Source: CAD feature listing. Evaluate the final solid. Frame: model axes, mm. A direction names the side the tool comes from. Give positions to 0.01 mm unless a question says otherwise; leave off trailing zeros. Loops run counter-clockwise (first coordinate to the right, second up) from the corner with the lowest first, then second, coordinate; pieces in that order, holes last.
```python
from build123d import *

# Parameters (mm, degrees)
SKETCH1_R            = 44.45
SKETCH1_R_2          = 36
BOSS_EXTRUDE1_DEPTH  = 3
SKETCH1_3_R          = 36
SKETCH1_3_R_2        = 32.5
BOSS_EXTRUDE2_DEPTH  = 2
M3_CLEARANCE_HOLE1_D = 3.2
CIRPATTERN1_COUNT    = 5


with BuildPart() as part:
    # Sketch1 → Boss-Extrude1 (new body)
    with BuildSketch(Plane(origin=(0, 0, 0), x_dir=(1, 0, 0), z_dir=(0, 1, 0))):
        with Locations(Location((0, 0, 0), (0, 0, 270))):
            Circle(SKETCH1_R)
        with Locations(Location((0, 0, 0), (0, 0, 270))):
            Circle(SKETCH1_R_2, mode=Mode.SUBTRACT)
    extrude(amount=BOSS_EXTRUDE1_DEPTH)

    # Sketch1_3 → Boss-Extrude2 (add)
    with BuildSketch(Plane(origin=(0, 0, 0), x_dir=(1, 0, 0), z_dir=(0, 1, 0))):
        with Locations(Location((0, 0, 0), (0, 0, 270))):
            Circle(SKETCH1_3_R)
        with Locations(Location((0, 0, 0), (0, 0, 270))):
            Circle(SKETCH1_3_R_2, mode=Mode.SUBTRACT)
    extrude(amount=BOSS_EXTRUDE2_DEPTH)

    # M3 Clearance Hole1 (through all)
    with Locations(Plane(origin=(0, 3, 0), x_dir=(1, 0, 0), z_dir=(0, 1, 0))):
        with Locations((-41.5, 0)):
            m3_clearance_hole1 = Hole(M3_CLEARANCE_HOLE1_D / 2)

    # CirPattern1: M3 Clearance Hole1 ×5 about axis
    cirpattern1_axis = Axis((0, 0, 0), (0, 1, 0))
    for i in range(1, CIRPATTERN1_COUNT):
        add(m3_clearance_hole1.rotate(cirpattern1_axis, i * 360 / CIRPATTERN1_COUNT), mode=Mode.SUBTRACT)


solid = part.part
```
(1) Section B-B, the plane z = 0. Return the cut outline in (x, y).
A:
outline: (-44.45, 0) - (-43.1, 0) - (-43.1, 3) - (-44.45, 3) - close; (-39.9, 0) - (-32.5, 0) - (-32.5, 2) - (-36, 2) - (-36, 3) - (-39.9, 3) - close; (32.5, 0) - (44.45, 0) - (44.45, 3) - (36, 3) - (36, 2) - (32.5, 2) - close
(2) Section C-C, the plane y = 2.5. Return the cut outline in (x, z).
A:
outline: circle Ø88.9 at (0, 0); hole circle Ø3.2 at (-41.5, 0); hole circle Ø72 at (0, 0); hole circle Ø3.2 at (-12.82, -39.47); hole circle Ø3.2 at (-12.82, 39.47); hole circle Ø3.2 at (33.57, -24.39); hole circle Ø3.2 at (33.57, 24.39)
(3) Ray query, line 1 along X through (y, z) = (0.85, 23); line 2 along X through (y, z) = (0.85, 25); line 3 along X through (y, z) = (2.25, -6.5). Return the intervals inside material, ascending.
A:
line 1: x = -38.04 to -22.96, 22.96 to 32.79, 34.36 to 38.04
line 2: x = -36.75 to -20.77, 20.77 to 32.09, 35.05 to 36.75
line 3: x = -43.97 to -35.41, 35.41 to 43.97
(4) Mould query, pull axis Z, two halves, no side actions, for faces 1 (the flat face through (-36, 3, -4)), 2 (the cylindrical face through (37.48, 1.48, 23.9)), 3 (the cylindrical face through (9.76, 0.99, 31)). Classes: pulls with the +Z half, pulls with the -Z half, needs draft (parallel to the pull), parting line crosses it, or undercut.
A:
face 1: needs draft
face 2: parting line crosses it
face 3: undercut
(5) First-contact query: pin 1 (1.5 mm diameter, centred on y = 1.5, z = 27.5, fed in from +X); pin 2 (1 mm diameter, centred on x = -11.5, y = 1.5, fed in from +Z). Flat tips, straight axial feed; report the tip coordinate or a pass-through.
A:
pin 1: stops at x = 35.5
pin 2: stops at z = 43.07
(6) Reachability of faces 4 (the cylindrical face through (10.81, 2.49, 34.34)), 5 (the cylindrical face through (-11.43, 1.48, -38.68)) from +Z, -Z, +X, -X, +Y, -Y: full face, straight path, thin tool, end or side. Return the list, or none.
A:
face 4: +Y
face 5: +Y, -Y
(7) Section A-A, the plane x = 0. Return the cut outline in (y, z), then the cut area to 3 significant figures.
A:
outline: (0, -44.45) - (3, -44.45) - (3, -36) - (2, -36) - (2, -32.5) - (0, -32.5) - close; (0, 32.5) - (2, 32.5) - (2, 36) - (3, 36) - (3, 44.45) - (0, 44.45) - close
area: 64.7 mm2
(8) Section D-D, the plane z = -21. Return the cut outline in (x, y).
A:
outline: (-39.18, 0) - (-24.8, 0) - (-24.8, 2) - (-29.24, 2) - (-29.24, 3) - (-39.18, 3) - close; (24.8, 0) - (39.18, 0) - (39.18, 3) - (29.24, 3) - (29.24, 2) - (24.8, 2) - close
